Can you work these out from the model? Positions are in its coordinate system, mm. Face numbers are marked on the shaded views. Round coordinates to 2 decimals unless told otherwise and drop trailing zeros. Write each loop counter-clockwise with the first axis right and the second up, starting at its lowest first coordinate (ties: lowest second). Pieces come first, ordered by that corner, then holes. Notation, with made-up numbers: (55.25, 50) -> (88.25, 50) arc R23 ccw to (88.25, 59) -> close; hole circle Ø5 at (36.25, 80.5). An arc over 180 degrees is marked (long way). Use CSV: the item, a comma, the result in double quotes.
Autodesk Inventor part; units mm, degrees
ref_plane "YZ Plane" through (0, 0, 0) normal (1, 0, 0) x (0, 1, 0)
ref_plane "XZ Plane" through (0, 0, 0) normal (0, 1, 0) x (-1, 0, 0)
ref_plane "XY Plane" through (0, 0, 0) normal (0, 0, 1) x (1, 0, 0)
sketch "Sketch1" plane through (0, 0, 0) normal (0, 0, 1) x (1, 0, 0)
  line L0 (0, 150) -> (129.9038, 75)
  line L1 (129.9038, 75) -> (129.9038, -75)
  line L2 (129.9038, -75) -> (0, -150)
  line L3 (0, -150) -> (-129.9038, -75)
  line L4 (-129.9038, -75) -> (-129.9038, 75)
  line L5 (-129.9038, 75) -> (0, 150)
  point P0 (0, 0)
  point P1 (0, 0)
  dimension "d0" = 150
extrude "Extrusion1" add sketch "Sketch1" along normal blind 2.5
sketch "Sketch2" plane through (0, 0, 2.5) normal (0, 0, 1) x (1, 0, 0)
  circle A0 centre (0, 0) radius 5
  dimension "d3" = 10
extrude "Extrusion2" cut sketch "Sketch2" against normal blind 10
sketch "Sketch3" plane through (0, 0, 2.5) normal (0, 0, 1) x (1, 0, 0)
  circle A0 centre (0, 0) radius 5
sheet face with bend "Face1" sketch "Sketch3" thickness 3.048 toward (0, 0, -1) bend radius 3.048
bend "Bend1"
equation "\"d6\" = Thickness"
equation "\"d7\" = BendRadius"
equation "\"d8\" = BendReliefWidth"
equation "\"d10\" = MinimumRemnant"
equation "\"d9\" = BendReliefDepth"
equation "\"d11\" = TransitionRadius"
equation "\"BendRadius\" = Thickness"
equation "\"BendReliefWidth\" = Thickness"
equation "\"BendReliefDepth\" = 0.5 * Thickness"
equation "\"CornerReliefSize\" = 4 * Thickness"
equation "\"MinimumRemnant\" = 2 * Thickness"
equation "\"TransitionRadius\" = BendRadius"
equation "\"JacobiRadiusSize\" = BendRadius"
equation "\"GapSize\" = Thickness"
properties part number "Bottom plate 2.5mm" material "Aluminum 6061"
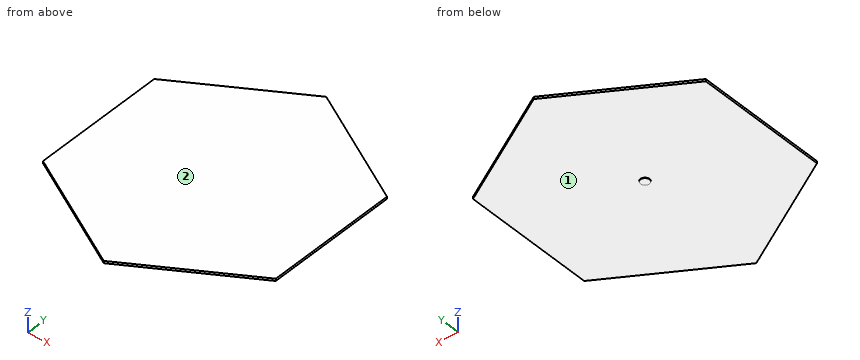
Q1. Please list where these lines run through material, in increasing order: probe 1 along Z at (x, y) = (37, 28); probe 2 along Y at (x, z) = (75, 1.8); probe 3 along X at (y, z) = (-121, 0.2).
Resolved:
probe 1,"z = 0 to 2.5"
probe 2,"y = -106.7 to 106.7"
probe 3,"x = -50.23 to 50.23"
Q2. Suppose I cut it at D-D (y = 31). Write out the boundary of the cut face in (x, z).
Resolved:
outline,"(-129.9, 0) -> (129.9, 0) -> (129.9, 2.5) -> (-129.9, 2.5) -> close"
Q3. Will these pins go through, and if not, where does the flat tip stop? P1, Ø2, axis at x = -3.5, y = 28, coming from the -Z side; P2, Ø1, axis at x = 55.5, z = 0, coming from the -Y side.
Resolved:
P1,"stops at z = 0"
P2,"stops at y = -118.25"
Q4. Suppose I cut it at A-A (y = 0). Write out the boundary of the cut face in (x, z).
Resolved:
outline,"(-129.9, 0) -> (-5, 0) -> (-5, -0.55) -> (5, -0.55) -> (5, 0) -> (129.9, 0) -> (129.9, 2.5) -> (-129.9, 2.5) -> close"
Q5. Suppose I cut it at C-C (x = 13.5). Write out the boundary of the cut face in (y, z).
Resolved:
outline,"(-142.21, 0) -> (142.21, 0) -> (142.21, 2.5) -> (-142.21, 2.5) -> close"
Q6. Suppose I cut it at B-B (z = 1.75). Write out the boundary of the cut face in (x, y).
Resolved:
outline,"(-129.9, -75) -> (0, -150) -> (129.9, -75) -> (129.9, 75) -> (0, 150) -> (-129.9, 75) -> close"
Q7. If we mould it in two halves opening along Z, with no side actions, what happens to the marked faces 1 and 2? For each: released by +Z, released by -Z, zero draft, split by the parting line, or undercut.
Resolved:
face 1,"released by -Z"
face 2,"released by +Z"
